Verification items for the finished model (mm, model axes). A direction names the side the tool comes from. Give positions to 0.01 mm unless a question says otherwise; leave off trailing zeros. Loops run counter-clockwise (first coordinate to the right, second up) from the corner with the lowest first, then second, coordinate; pieces in that order, holes last. Notation, with made-up numbers: M -26,66.25 L -5,66.25 A14 cw -5,93.25 Z; hole C -13.5,47.5 d8. An arc over 180 degrees is marked long. Answer in a Markdown table with one row per item.
Autodesk Inventor part; units mm, degrees
ref_plane "YZ Plane" through (0, 0, 0) normal (1, 0, 0) x (0, 1, 0)
ref_plane "XZ Plane" through (0, 0, 0) normal (0, 1, 0) x (-1, 0, 0)
ref_plane "XY Plane" through (0, 0, 0) normal (0, 0, 1) x (1, 0, 0)
sketch "Sketch1" plane through (0, 0, 0) normal (0, 0, 1) x (1, 0, 0)
  line L0 (-21, 26) -> (21, 26)
  line L1 (21, 26) -> (21, -26)
  line L2 (21, -26) -> (-21, -26)
  line L3 (-21, -26) -> (-21, 26)
  line L4 (-21, 26) -> (21, -26) construction
  line L5 (21, 26) -> (-21, -26) construction
  line L6 (-15.5, 20.5) -> (15.5, -20.5) construction
  line L7 (15.5, 20.5) -> (-15.5, -20.5) construction
  line L8 (-11.5, -5) -> (-11.5, 5)
  line L9 (11.5, -5) -> (11.5, 5)
  arc A0 (4.507, 5.58) -> (4.2877, 5.6708) centre (0, -5) ccw
  arc A1 (-4.2877, 5.6708) -> (-4.507, 5.58) centre (0, -5) ccw
  arc A2 (-11.5, -5) -> (11.5, -5) centre (0, -5) ccw
  arc A3 (-4.507, -5.58) -> (-4.2877, -5.6708) centre (0, 5) ccw
  arc A4 (4.2877, -5.6708) -> (4.507, -5.58) centre (0, 5) ccw
  arc A5 (11.5, 5) -> (-11.5, 5) centre (0, 5) ccw
  line L10 (-15.5, -20.5) -> (-15.5, -10.5)
  arc A6 (-13.75, -10.5) -> (-17.25, -10.5) centre (-15.5, -10.5) ccw
  line L11 (-13.75, -20.5) -> (-13.75, -10.5)
  line L12 (-17.25, -10.5) -> (-17.25, -20.5)
  arc A7 (-17.25, -20.5) -> (-13.75, -20.5) centre (-15.5, -20.5) ccw
  arc A8 (17.25, -10.5) -> (13.75, -10.5) centre (15.5, -10.5) ccw
  line L13 (17.25, -20.5) -> (17.25, -10.5)
  line L14 (13.75, -10.5) -> (13.75, -20.5)
  arc A9 (13.75, -20.5) -> (17.25, -20.5) centre (15.5, -20.5) ccw
  arc A10 (-13.75, 20.5) -> (-17.25, 20.5) centre (-15.5, 20.5) ccw
  line L15 (-13.75, 10.5) -> (-13.75, 20.5)
  line L16 (-17.25, 20.5) -> (-17.25, 10.5)
  arc A11 (-17.25, 10.5) -> (-13.75, 10.5) centre (-15.5, 10.5) ccw
  arc A12 (17.25, 20.5) -> (13.75, 20.5) centre (15.5, 20.5) ccw
  line L17 (17.25, 10.5) -> (17.25, 20.5)
  line L18 (13.75, 20.5) -> (13.75, 10.5)
  arc A13 (13.75, 10.5) -> (17.25, 10.5) centre (15.5, 10.5) ccw
  point P0 (0, 0)
  dimension "d0" = 42
  dimension "d1" = 52
  dimension "d2" = 31
  dimension "d3" = 41
  dimension "d9" = 5
  dimension "d10" = 5
  dimension "d12" = 10
  dimension "d13" = 3.5
  dimension "d14" = 3.5
  dimension "d15" = 3.5
  dimension "d16" = 3.5
  dimension "d17" = 20.5
  dimension "d18" = 20.5
  dimension "d19" = 20.5
  dimension "d20" = 20.5
extrude "Extrusion1" add sketch "Sketch1" along normal blind 3
sketch "Sketch2" plane through (-21, 26, 0) normal (0, 1, 0) x (1, 0, 0)
  line L0 (42, -3) -> (0, -3)
  line L1 (0, -3) -> (42, -3)
  line L2 (42, -3) -> (42, 10)
  line L3 (42, 10) -> (0, 10)
  line L4 (0, 10) -> (0, -3)
  point P0 (21, 0)
  dimension "d23" = 13
extrude "Extrusion2" add sketch "Sketch2" along normal blind 3
sketch "Sketch3" plane through (21, 26, -10) normal (0, 0, -1) x (-1, 0, 0)
  line L0 (42, 0) -> (0, 0)
  line L1 (42, 0) -> (0, 0)
  line L2 (0, 0) -> (0, 23)
  line L3 (0, 23) -> (42, 23)
  line L4 (42, 23) -> (42, 0)
  point P0 (21, -26)
  dimension "d26" = 23
extrude "Extrusion3" add sketch "Sketch3" along normal blind 6
sketch "Sketch6" plane through (21, 26, -10) normal (0, 0, 1) x (1, 0, 0)
  point P0 (-21, -26)
  point P1 (-10.5, 13)
  point P2 (-31.5, 13)
sketch "Sketch7" plane through (21, 26, -16) normal (0, 0, -1) x (-1, 0, 0)
  circle A0 centre (31.5, 13) radius 2.75
  circle A1 centre (10.5, 13) radius 2.75
  line L0 (42, 10) -> (0, 10)
  line L1 (42, 16) -> (0, 16)
  line L2 (42, 0) -> (42, 23)
  line L3 (42, 0) -> (42, 23)
  line L4 (0, 0) -> (42, 0)
  line L5 (0, 3) -> (0, 23)
  line L6 (0, 0) -> (0, 23)
  point P0 (21, -26)
extrude "Extrusion4" add sketch "Sketch7" along normal blind 1.5 contours L0 L5 L1 L2
sketch "Sketch8" plane through (21, 26, -17.5) normal (0, 0, -1) x (-1, 0, 0)
  circle A0 centre (31.5, 13) radius 2.75
  circle A1 centre (10.5, 13) radius 2.75
  point P0 (21, -26)
hole "Hole2" at (-10.5, 39, -17.5) at (10.5, 39, -17.5) direction (0, 0, 1) diameter 5.5 end through all counterbore diameter 10 counterbore depth 1.5
chamfer "Chamfer2" distance 3 angle 45 2 edges at (0, 26, 0) (0, 29, -10)
properties part number "Suporte Z Motor"
Item 1: Sectioned sample at C-C (z = -14.25). Record the cut outline in (x, y), and give its area (3 significant figures).
Reported:
| item | result |
|---|---|
| outline | M -21,26 L 21,26 L 21,49 L -21,49 Z; hole C -10.5,39 d5.5; hole C 10.5,39 d5.5 |
| area | 918 mm^2 |
Item 2: Release check for a two-part mould opening along X. For faces 5 (the flat face through (-21, 20, 0.4)), 6 (the cylindrical face through (-15.46, -22.25, 1.48)), 7 (the flat face through (14, -1, 0)) record: released by +X, released by -X, zero draft, split by the parting line, or undercut.
Reported:
| item | result |
|---|---|
| face 5 | released by -X |
| face 6 | undercut |
| face 7 | zero draft |
Item 3: Scan lines: L1, parallel to X at y = 39, z = -12.95; L2, parallel to Y at x = -10.5, z = -13.25; L3, parallel to Y at x = 18.5, z = -3.25. Record each from-to range of solid material in increasing order. Write a range as [from, to].
Reported:
| item | result |
|---|---|
| L1 | x = [-21, -13.25], [-7.75, 7.75], [13.25, 21] |
| L2 | y = [26, 36.25], [41.75, 49] |
| L3 | y = [26, 29] |
Item 4: Go/stop test with flat-tipped pins: pin 1 (12 mm diameter, centred on y = 9.5, z = -9, fed in from +X); pin 2 (4 mm diameter, centred on x = -11, y = 5.5, fed in from -Z); pin 3 (1.2 mm diameter, centred on x = 19, z = -16.5, fed in from -Y); pin 4 (9 mm diameter, centred on x = -10.5, y = 39, fed in from -Z). Record where each tip stops, or that it passes through.
Reported:
| item | result |
|---|---|
| pin 1 | passes through |
| pin 2 | stops at z = 0 |
| pin 3 | stops at y = 26 |
| pin 4 | stops at z = -16 |
Item 5: Sectioned sample at D-D (x = 18.5). Record the cut outline in (y, z).
Reported:
| item | result |
|---|---|
| outline | M -26,0 L 23,0 L 26,-3 L 26,-16 L 36,-16 L 36,-17.5 L 42,-17.5 L 42,-16 L 49,-16 L 49,-10 L 32,-10 L 29,-7 L 29,3 L -26,3 Z |
Item 6: Sectioned sample at B-B (x = 10.5). Record the cut outline in (y, z).
Reported:
| item | result |
|---|---|
| outline | M -26,0 L -9.69,0 L -9.69,3 L -26,3 Z; M 9.69,0 L 23,0 L 26,-3 L 26,-16 L 36.25,-16 L 36.25,-10 L 32,-10 L 29,-7 L 29,3 L 9.69,3 Z; M 41.75,-16 L 49,-16 L 49,-10 L 41.75,-10 Z |
Item 7: Tool access check on faces 1 (the flat face through (18, 42, -17)), 2 (the flat face through (0, 36, -17)), 3 (the flat face through (0, 41, -10)), 4 (the cylindrical face through (15.54, -22.25, 1.48)). Record the directions out of +Z, -Z, +X, -X, +Y, -Y that give a thin tool (end or side, any length) a straight path to the whole face; none if there is none.
Reported:
| item | result |
|---|---|
| face 1 | -Z, +X, -X, +Y |
| face 2 | -Z, +X, -X, -Y |
| face 3 | +Z, +X, -X, +Y |
| face 4 | +Z, -Z |
Item 8: Sectioned sample at A-A (y = -17.5). Record the cut outline in (x, z).
Reported:
| item | result |
|---|---|
| outline | M -21,0 L -17.25,0 L -17.25,3 L -21,3 Z; M -13.75,0 L 13.75,0 L 13.75,3 L -13.75,3 Z; M 17.25,0 L 21,0 L 21,3 L 17.25,3 Z |
